Part print with two shaded views. Sizes in mm from the minimum x, y, z corner. A direction names the side the tool comes from. Coordinates: 2 decimals unless noted, no trailing zeros. Write each loop counter-clockwise with the first axis right and the second up, starting at its lowest first coordinate (ties: lowest second). Pieces come first, ordered by that corner, then holes. Notation, with made-up numbers: M 45.5,49 L 95.5,49 A26 ccw 95.5,65 Z; hole C 74.5,-23.75 d9. An arc over 180 degrees is marked long. Use CSV: the item, a comma, the result in double quotes. Start each with the question number.
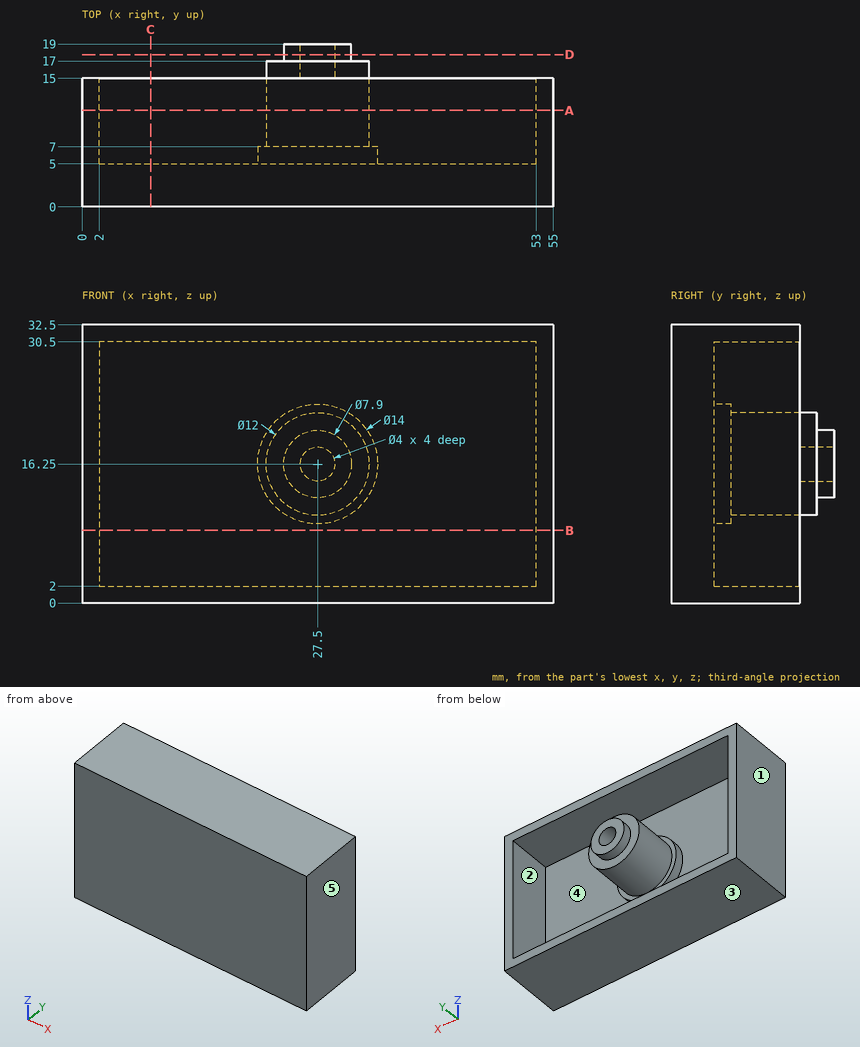
1. Flat gauge pins, fed straight in: pin 1 (1.5 mm diameter, centred on x = 26, z = 10.5, fed in from -Y); pin 2 (8 mm diameter, centred on x = 47.5, z = 14.5, fed in from +Y); pin 3 (1.2 mm diameter, centred on x = 28, z = 15.5, fed in from +Y). Where does each tip first touch, or does it go through?
2. Drill centre lines: line 1 along Z through (x, y) = (27.5, 16.8); line 2 along X through (y, z) = (15.9, 16.25); line 3 along Z through (x, y) = (5, 5.25). Where is each one in solid material? Low to high. Write a range as from..to.
3. Slice it at B-B (z = 8.5). List the corners of the cut face in (x, y).
4. 3-axis set-ups, long thin cutter, end or side, ignore diameter. For the marked faces 1 and 2: which of +Z, -Z, +X, -X, +Y, -Y reach the whole face in a straight line?
5. Slice it at A-A (y = 11.25). List the corners of the cut face in (x, z), and give its area (3 significant figures).
6. Pull direction Z, two halves, no side cores. Call the marked faces 3, 4 and 5: pulls with the +Z half, pulls with the -Z half, needs draft (parallel to the pull), parting line crosses it, or undercut.
7. Slice it at C-C (x = 8). List the corners of the cut face in (y, z), and give its area (4 significant figures).
8. Slice it at D-D (y = 17.75). List the corners of the cut face in (x, z), and give its area (3 significant figures).
Established:
1,pin 1,"stops at y = 0"
1,pin 2,"stops at y = 5"
1,pin 3,"stops at y = 15"
2,line 1,"z = 10.25..14.25, 18.25..22.25"
2,line 2,"x = 21.5..25.5, 29.5..33.5"
2,line 3,"z = 0..2, 30.5..32.5"
3,outline,"M 0,0 L 55,0 L 55,15 L 53,15 L 53,5 L 2,5 L 2,15 L 0,15 Z"
4,face 1,"+Z, -Z, -X, +Y, -Y"
4,face 2,"+Y"
5,outline,"M 0,0 L 55,0 L 55,32.5 L 0,32.5 Z; C 27.5,16.25 d12; hole M 2,2 L 53,2 L 53,30.5 L 2,30.5 Z"
5,area,"447 mm2"
6,face 3,"pulls with the -Z half"
6,face 4,"undercut"
6,face 5,"needs draft"
7,outline,"M 0,0 L 15,0 L 15,2 L 5,2 L 5,30.5 L 15,30.5 L 15,32.5 L 0,32.5 Z"
7,area,"202.5 mm2"
8,outline,"C 27.5,16.25 d7.9; hole C 27.5,16.25 d4"
8,area,"36.5 mm2"
